Verification items for the finished model (mm, model axes). A direction names the side the tool comes from. Give positions to 0.01 mm unless a question says otherwise; leave off trailing zeros. Loops run counter-clockwise (first coordinate to the right, second up) from the corner with the lowest first, then second, coordinate; pieces in that order, holes last. Notation, with made-up numbers: (27, -5.75) - (60, -5.75) arc R31 cw to (60, 18.25) - close; hole circle Ø9 at (18.25, 60). An arc over 180 degrees is marked (long way). One line per question, with ' | ' between items. Start each with the question number.
1. Section check A-A, the plane y = -10. Enter the section's corners in (x, z).
2. Tool access check on faces 1 (the face through (4.868, 56.79, 53.651)), 2 (the face through (40, 21, -1)), 3 (the face through (0, -11, 65)), 4 (the face through (75, -9, 1)). Record the directions out of +Z, -Z, +X, -X, +Y, -Y that give a thin tool (end or side, any length) a straight path to the whole face; none if there is none.
3. Thickness scan on line 1 along X through (y, z) = (57, -60); line 2 along Z through (x, y) = (0, 62); line 3 along Z through (x, y) = (0, -8.75). Record the ranges inside material, lowest first. Write a range as from..to.
4. Section check B-B, the plane x = -49.5. Enter the section's corners in (y, z), then the cut area to 3 significant figures.
5. Section check C-C, the plane y = 49. State how many separate pieces and enclosed holes the cut face has, then the cut area to 3 significant figures.
6. Mould release check, pull along Z, two halves, no side actions. Record for faces 5 (the face through (59.152, -1.533, 0.188)), 6 (the face through (-75, -9, -1)), 7 (the face through (-1, 21, -40)): +Z half, -Z half, draft (parallel to the pull), parting line (faces both ways), or undercut.
7. Depth check by flat-ended pin: pin 1 Ø6 at (x, z) = (0, 60) entering from -Y; pin 2 Ø13 at (x, z) = (60, 0) entering from +Y; pin 3 Ø16 at (x, z) = (0, 0) entering from +Y; pin 4 Ø1.5 at (y, z) = (20, -22) entering from +X. Enter the tip coordinate at first touch or a pass-through.
8. Section check D-D, the plane z = -34.5. Enter the section's corners in (x, y).
Autodesk Inventor part; units mm, degrees
ref_plane "YZ Plane" through (0, 0, 0) normal (1, 0, 0) x (0, 1, 0)
ref_plane "XZ Plane" through (0, 0, 0) normal (0, 1, 0) x (-1, 0, 0)
ref_plane "XY Plane" through (0, 0, 0) normal (0, 0, 1) x (1, 0, 0)
sketch "Sketch1" plane through (0, 0, 0) normal (0, 1, 0) x (-1, 0, 0)
  line L0 (-75, -75) -> (75, -75)
  line L1 (75, -75) -> (75, 75)
  line L2 (75, 75) -> (-75, 75)
  line L3 (-75, 75) -> (-75, -75)
  line L4 (-75, -75) -> (75, 75) construction
  line L5 (75, -75) -> (-75, 75) construction
  point P0 (0, 0)
  dimension "d0" = 150
  dimension "d1" = 150
extrude "Extrusion1" add sketch "Sketch1" against normal blind 18
sketch "Sketch2" plane through (0, -18, 0) normal (0, -1, 0) x (1, 0, 0)
  circle A0 centre (0, 0) radius 30
  line L0 (-60, -60) -> (60, -60) construction
  line L1 (60, -60) -> (60, 60) construction
  line L2 (60, 60) -> (-60, 60) construction
  line L3 (-60, 60) -> (-60, -60) construction
  line L4 (-60, -60) -> (60, 60) construction
  line L5 (60, -60) -> (-60, 60) construction
  dimension "d4" = 60
  dimension "d5" = 120
  dimension "d6" = 120
extrude "Extrusion2" cut sketch "Sketch2" against normal blind 10
sketch "Sketch3" plane through (0, -18, 0) normal (0, -1, 0) x (1, 0, 0)
  line L0 (60, -60) -> (60, 60) construction
  line L1 (60, 60) -> (-60, 60) construction
  line L2 (-60, 60) -> (-60, -60) construction
  line L3 (-60, -60) -> (60, -60) construction
  point P0 (0, 0)
  point P1 (60, 0)
  point P2 (-60, 0)
  point P3 (0, 60)
  point P4 (0, -60)
hole "Hole1" at (0, -18, 60) at (-60, -18, 0) at (0, -18, -60) at (60, -18, 0) direction (0, 1, 0) diameter 10 depth 13 tip angle 100
sketch "Sketch4" plane through (0, 0, 0) normal (0, 1, 0) x (1, 0, 0)
  line L0 (40, -40) -> (-40, -40)
  line L1 (-40, -40) -> (-40, 40)
  line L2 (-40, 40) -> (40, 40)
  line L3 (40, 40) -> (40, -40)
  line L4 (40, -40) -> (-40, 40) construction
  line L5 (-40, -40) -> (40, 40) construction
  point P0 (0, 0)
  dimension "d16" = 80
  dimension "d17" = 80
extrude "Extrusion3" add sketch "Sketch4" along normal blind 42
sketch "Sketch5" plane through (0, 42, 0) normal (0, 1, 0) x (1, 0, 0)
  line L0 (75, -75) -> (-75, -75)
  line L1 (-75, -75) -> (-75, 75)
  line L2 (-75, 75) -> (75, 75)
  line L3 (75, 75) -> (75, -75)
  line L4 (75, -75) -> (-75, 75) construction
  line L5 (-75, -75) -> (75, 75) construction
  point P0 (0, 0)
extrude "Extrusion4" add sketch "Sketch5" along normal blind 30
sketch "Sketch6" plane through (0, 72, 0) normal (0, 1, 0) x (1, 0, 0)
  circle A0 centre (0, 0) radius 13.5
  dimension "d22" = 27
extrude "Extrusion5" cut sketch "Sketch6" against normal through all
sketch "Sketch7" plane through (0, 72, 0) normal (0, 1, 0) x (1, 0, 0)
  line L0 (60, 60) -> (-60, 60) construction
  line L1 (-60, 60) -> (-60, -60) construction
  line L2 (-60, -60) -> (60, -60) construction
  line L3 (60, -60) -> (60, 60) construction
  line L4 (60, 60) -> (-60, -60) construction
  line L5 (-60, 60) -> (60, -60) construction
  point P0 (0, 0)
  point P1 (0, 60)
  point P2 (-60, 0)
  point P3 (0, -60)
  point P4 (60, 0)
  dimension "d25" = 120
  dimension "d26" = 120
hole "Hole2" at (-60, 72, 60) at (0, 72, 60) at (60, 72, 60) at (60, 72, 0) at (60, 72, -60) at (0, 72, -60) at (-60, 72, -60) at (-60, 72, 0) direction (0, -1, 0) diameter 16 depth 30
thread "Thread2"
thread "Thread3"
thread "Thread4"
thread "Thread5"
thread "Thread6"
thread "Thread7"
thread "Thread8"
thread "Thread9"
properties material "Iron, Cast"
Results list:
1) outline: (-75, -75) - (75, -75) - (75, 75) - (-75, 75) - close; hole circle Ø10 at (-60, 0); hole circle Ø60 at (0, 0); hole circle Ø10 at (0, -60); hole circle Ø10 at (0, 60); hole circle Ø10 at (60, 0)
2) face 1: +Y | face 2: +Z, -Z, +X | face 3: -Y | face 4: +Z, -Z, +X, +Y, -Y
3) line 1: -75..-68, -52..-8, 8..52, 68..75 | line 2: -75..-68, -52..-13.5, 13.5..52, 68..75 | line 3: -75..-65, -55..-30, 30..55, 65..75
4) outline: (-18, -75) - (0, -75) - (0, 75) - (-18, 75) - close; (42, -75) - (72, -75) - (72, 75) - (42, 75) - close | area: 7,200 mm²
5) separate pieces: 1 | enclosed holes: 9 | area: 20,300 mm²
6) face 5: undercut | face 6: draft | face 7: -Z half
7) pin 1: y = -3.32 | pin 2: y = 0 | pin 3: through | pin 4: x = 40
8) outline: (-75, -18) - (75, -18) - (75, 0) - (40, 0) - (40, 42) - (75, 42) - (75, 72) - (-75, 72) - (-75, 42) - (-40, 42) - (-40, 0) - (-75, 0) - close
